```python
from build123d import *

# Parameters (mm, degrees)
F0_W     = 6.3
F0_H     = 6.3
F0_R     = 1.6
F1_DEPTH = 0.2
F2_W     = 0.2
F2_H     = 6.3
F3_DEPTH = 1.8
F4_R     = 0.2


with BuildPart() as f1:
    # F0 (on Top) → F1 (new body)
    with BuildSketch(Plane.XY):
        with Locations((3.15, 3.15)):
            Rectangle(F0_W, F0_H)
        with Locations((3.15, 3.15)):
            Circle(F0_R, mode=Mode.SUBTRACT)
    extrude(amount=F1_DEPTH)

    # F2 (on face) → F3 (join)
    with BuildSketch(Plane(origin=(0, 0, 0), x_dir=(1, 0, 0), z_dir=(0, 0, -1))):
        with Locations((0.1, -3.15)):
            Rectangle(F2_W, F2_H)
        with Locations((6.2, -3.15)):
            Rectangle(F2_W, F2_H)
    extrude(amount=F3_DEPTH)

    # F4
    f4_edges = [f1.edges().sort_by_distance(p)[0] for p in [
        (0, 3.15, 0.2),
        (6.3, 3.15, 0.2),
    ]]
    fillet(f4_edges, radius=F4_R)


solid = f1.part
```
Model file for the job. Use its own axes, mm. Coordinates: 2 decimals unless noted, no trailing zeros. Write each loop counter-clockwise with the first axis right and the second up, starting at its lowest first coordinate (ties: lowest second). Pieces come first, ordered by that corner, then holes. Notation, with made-up numbers: (-30.75, -20.5) - (27.25, -20.5) arc R15 cw to (27.25, -10.5) - close; hole circle Ø1 at (32.5, 15). An arc over 180 degrees is marked (long way). Use a Markdown table: item, result. Add a question column.
Item 1: Band-saw the part on B-B, the plane x = 3.15. Write the cut outline in (y, z).
Item 2: Band-saw the part on A-A, the plane z = -1.6. Write the cut outline in (x, y), and give its area (3 significant figures).
Item 3: Band-saw the part on C-C, the plane y = 3.15. Write the cut outline in (x, z), and give its area (3 significant figures).
Item 4: Band-saw the part on D-D, the plane y = 1. Write the cut outline in (x, z).
Item 5: Drill centre lines: line 1 along Y through (x, z) = (3.15, 0.1); line 2 along X through (y, z) = (1.5, -0.15); line 3 along Z through (x, y) = (4.5, 5). Where is each one in solid material? Low to high.
Item 6: Drop a flat-ended pin along its axis: pin 1 (1.5 mm diameter, centred on x = 4, y = 4.5, fed in from -Z). Give the stop position or say it passes through.
Item 7: Two-plate mould, pull along X, no slides. Class faces 1 (the face through (0, 3, -1)), 2 (the face through (2, 5, 0.2)), 3 (the face through (0.2, 3, -1)), 4 (the face through (6.3, 3, -1)): pulls with the +X half, pulls with the -X half, needs draft (parallel to the pull), parting line crosses it, or undercut.
A:
| question | item | result |
|---|---|---|
| 1 | outline | (0, 0) - (1.55, 0) - (1.55, 0.2) - (0, 0.2) - close; (4.75, 0) - (6.3, 0) - (6.3, 0.2) - (4.75, 0.2) - close |
| 2 | outline | (0, 0) - (0.2, 0) - (0.2, 6.3) - (0, 6.3) - close; (6.1, 0) - (6.3, 0) - (6.3, 6.3) - (6.1, 6.3) - close |
| 2 | area | 2.52 mm² |
| 3 | outline | (0, -1.8) - (0.2, -1.8) - (0.2, 0) - (1.55, 0) - (1.55, 0.2) - (0.2, 0.2) arc R0.2 ccw to (0, 0) - close; (4.75, 0) - (6.1, 0) - (6.1, -1.8) - (6.3, -1.8) - (6.3, 0) arc R0.2 ccw to (6.1, 0.2) - (4.75, 0.2) - close |
| 3 | area | 1.32 mm² |
| 4 | outline | (0, -1.8) - (0.2, -1.8) - (0.2, 0) - (6.1, 0) - (6.1, -1.8) - (6.3, -1.8) - (6.3, 0) arc R0.2 ccw to (6.1, 0.2) - (0.2, 0.2) arc R0.2 ccw to (0, 0) - close |
| 5 | line 1 | y = 0 to 1.55, 4.75 to 6.3 |
| 5 | line 2 | x = 0 to 0.2, 6.1 to 6.3 |
| 5 | line 3 | z = 0 to 0.2 |
| 6 | pin 1 | stops at z = 0 |
| 7 | face 1 | pulls with the -X half |
| 7 | face 2 | needs draft |
| 7 | face 3 | undercut |
| 7 | face 4 | pulls with the +X half |
